Geometry: final body of the model. Coordinates: model frame, mm. A direction names the side the tool comes from. Round coordinates to 2 decimals unless told otherwise and drop trailing zeros. Loops run counter-clockwise (first coordinate to the right, second up) from the corner with the lowest first, then second, coordinate; pieces in that order, holes last. Notation, with made-up numbers: M -22.5,40.25 L 14.5,40.25 A19 ccw 14.5,61.25 Z; hole C 6.25,-18 d9. An arc over 180 degrees is marked long. Answer as a JSON object with one key per item and string values.
from build123d import *

# Parameters (mm, degrees)
SKETCH1_R           = 4.953
BOSS_EXTRUDE1_DEPTH = 25.4
FILLET1_R           = 12.7
FILLET2_R           = 2.54
CUT_EXTRUDE3_REACH  = 130.474
SKETCH5_R           = 5.08
CUT_EXTRUDE4_REACH  = 120.723
SKETCH7_R           = 3.175


with BuildPart() as part:
    # Sketch1 → Boss-Extrude1 (new body)
    with BuildSketch(Plane(origin=(0, 0, 0), x_dir=(0, 0, -1), z_dir=(1, 0, 0))):
        with BuildLine():
            Line((103.901886641, 61.637766497), (113.279686218, 73.483555297))
            Line((113.279686218, 73.483555297), (98.451355982, 83.391276702))
            Line((98.451355982, 83.391276702), (48.882530567, 82.21455605))
            Line((48.882530567, 82.21455605), (1.911791408, 41.210560809))
            Line((1.911791408, 41.210560809), (-8.886551045, -4.469459574))
            Line((-8.886551045, -4.469459574), (26.146598357, -19.557154557))
            ThreePointArc((26.146598357, -19.557154557), (36.159220082, -15.57265883), (32.174724356, -5.560037105))
            Line((32.174724356, -5.560037105), (8.886551045, 4.469459574))
            Line((8.886551045, 4.469459574), (15.618065001, 32.945653592))
            Line((15.618065001, 32.945653592), (54.753455571, 67.109633069))
            Line((54.753455571, 67.109633069), (94.084630156, 68.043320825))
            Line((94.084630156, 68.043320825), (103.901886641, 61.637766497))
        make_face()
        with Locations((3.213640173, 1.616289015)):
            Circle(SKETCH1_R, mode=Mode.SUBTRACT)
    extrude(amount=BOSS_EXTRUDE1_DEPTH)

    # Fillet1
    fillet1_edges = [part.edges().sort_by_distance(p)[0] for p in [
        (12.7, 68.043320825, -94.084630156),
        (12.7, 67.109633069, -54.753455571),
        (12.7, 32.945653592, -15.618065001),
        (12.7, 4.469459574, -8.886551045),
        (12.7, -4.469459574, 8.886551045),
        (12.7, 41.210560809, -1.911791408),
        (12.7, 82.21455605, -48.882530567),
        (12.7, 83.391276702, -98.451355982),
    ]]
    fillet(fillet1_edges, radius=FILLET1_R)

    # Fillet2
    fillet2_edges = [part.edges().sort_by_distance(p)[0] for p in [
        (12.7, 73.483555297, -113.279686218),
        (12.7, 61.637766497, -103.901886641),
    ]]
    fillet(fillet2_edges, radius=FILLET2_R)

    # Sketch5 → Cut-Extrude3 (cut, up to next)
    with BuildSketch(Plane(origin=(0, -6.998558726, 3.014062999), x_dir=(1, 0, 0), z_dir=(0, -0.918446027, 0.395546325)), mode=Mode.PRIVATE) as cut_extrude3_sk1:
        with Locations((12.7, -24.13)):
            Circle(SKETCH5_R)
    cut_extrude3_tool1 = extrude(cut_extrude3_sk1.sketch, amount=-CUT_EXTRUDE3_REACH, mode=Mode.PRIVATE) & part.part
    add(cut_extrude3_tool1.solids().sort_by_distance((12.7, -16.543092, -19.14804))[0], mode=Mode.SUBTRACT)

    # Sketch7 → Cut-Extrude4 (cut, up to next)
    with BuildSketch(Plane(origin=(0, 22.440379915, 19.589754126), x_dir=(1, 0, 0), z_dir=(0, 0.753334468, 0.657637574)), mode=Mode.PRIVATE) as cut_extrude4_sk1:
        with Locations((12.7, 45.316910599)):
            Circle(SKETCH7_R)
    cut_extrude4_tool1 = extrude(cut_extrude4_sk1.sketch, amount=-CUT_EXTRUDE4_REACH, mode=Mode.PRIVATE) & part.part
    add(cut_extrude4_tool1.solids().sort_by_distance((12.7, 52.242483, -14.549037))[0], mode=Mode.SUBTRACT)


solid = part.part
1) Section query B-B (z = -56). Return the cut outline in (x, y), and give its area (3 significant figures).
Results:
{"outline": "M 0,66.69 L 25.4,66.69 L 25.4,82.38 L 0,82.38 Z", "area": "399 mm2"}
2) Pin query (flat end, axial travel): P1, Ø1.5, axis at x = 13.5, y = 37.5, coming from the -Z side; P2, Ø10, axis at y = 33.5, z = -30.5, coming from the -X side; P3, Ø3, axis at x = 8, z = -44, coming from the +Y side; P4, Ø6, axis at x = 6, y = 39.5, coming from the -Z side. Return the tip coordinate at first contact, or that it passes through.
Results:
{"P1": "z = -21.69", "P2": "through", "P3": "y = 79.26", "P4": "z = -26.56"}
3) Section query C-C (y = 21). Return the cut outline in (x, z).
Results:
{"outline": "M 0,-12.79 L 25.4,-12.79 L 25.4,2.87 L 0,2.87 Z"}
4) Section query A-A (x = 19.25). Return the cut outline in (y, z) (1 decimal).
Results:
{"outline": "M -19.6,-26.1 A7.6 ccw -5.6,-32.2 L 0.3,-18.7 A12.7 cw 14.8,-11.3 L 29,-14.7 A12.7 cw 35.6,-18.7 L 64.1,-51.3 A12.7 cw 67.2,-59.3 L 67.9,-90.1 A12.7 cw 65.9,-97.4 L 62.9,-102 A2.5 ccw 63.5,-105.3 L 71.3,-111.6 A2.5 ccw 75,-111 L 81.2,-101.8 A12.7 ccw 83.3,-94.4 L 82.3,-53.5 A12.7 ccw 79.2,-45.4 L 43.9,-5 A12.7 ccw 37.2,-1 L 5.9,6.4 A12.7 ccw -8.7,-0.9 Z; hole C 1.6,-3.2 d9.9"}
5) Reachability of faces 4 (the cylindrical face through (12.878, -2.616, 5.477)), 5 (the cylindrical face through (12.88, 32.66, -16.19)), 6 (the flat face through (12.52, 64.42, -99.64)) from +Z, -Z, +X, -X, +Y, -Y: full face, straight path, thin tool, end or side. Return the list, or none.
Results:
{"face 4": "+Z, +X, -X", "face 5": "-Z, +X, -X", "face 6": "+X, -X, -Y"}
6) Pull-direction query (Z, two-part tool) for faces 1 (the cylindrical face through (12.039, -7.65, -17.494)), 2 (the cylindrical face through (12.878, 73.267, -112.093)), 3 (the cylindrical face through (12.52, -15.73, -36.09)); classes: +Z half, -Z half, draft (parallel to the pull), parting line (faces both ways), or undercut.
Results:
{"face 1": "undercut", "face 2": "-Z half", "face 3": "parting line"}
7) Ray query, line 1 (Y direction, x = 13.25, z = -17.5); line 2 (Y direction, x = 17.75, z = -15.5); line 3 (Z direction, x = 17.5, y = 6). Return the intervals inside material, ascending.
Results:
{"line 1": "-7.6 to 0.83, 34.44 to 44.11, 53.62 to 54.82", "line 2": "-14.97 to 2.22, 31.36 to 53.07", "line 3": "-12.46 to -5.52, -0.91 to 6.41"}
